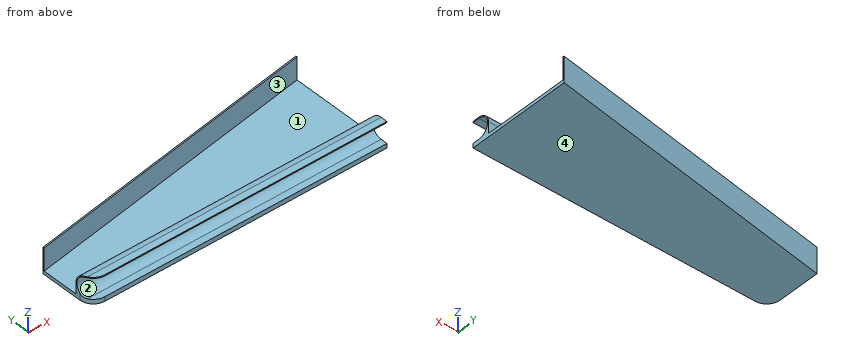
```python
from build123d import *

# Parameters (mm, degrees)
BOSS_EXTRUDE1_DEPTH     = 6.35
BOSS_EXTRUDE7_DEPTH     = 558.8
CUT_EXTRUDE1_DEPTH      = 551.191074589
CUT_EXTRUDE1_DEPTH_BACK = 551.191074589
BOSS_EXTRUDE8_DEPTH     = 42.164
CUT_EXTRUDE2_DEPTH      = 110.49


with BuildPart() as part:
    # Sketch1 → Boss-Extrude1 (new body)
    with BuildSketch(Plane.XY):
        with BuildLine():
            Line((-508.085110878, -34.117945662), (-508.085110878, -168.737945662))
            Line((-508.085110878, -168.737945662), (-508.085110878, -181.437945662))
            ThreePointArc((-508.085110878, -181.437945662), (-500.64562312, -199.398457904), (-482.685110878, -206.837945662))
            Line((-482.685110878, -206.837945662), (50.714889122, -206.837945662))
            Line((50.714889122, -206.837945662), (50.714889122, -8.717945662))
            Line((50.714889122, -8.717945662), (-482.685110878, -8.717945662))
            ThreePointArc((-482.685110878, -8.717945662), (-500.64562312, -16.15743342), (-508.085110878, -34.117945662))
        make_face()
    extrude(amount=BOSS_EXTRUDE1_DEPTH)

    # Sketch3 → Boss-Extrude7 (add)
    with BuildSketch(Plane(origin=(50.714889122, 0, 0), x_dir=(0, 0, -1), z_dir=(1, 0, 0))):
        with BuildLine():
            Line((-6.35, -173.055945662), (-27.432, -173.055945662))
            ThreePointArc((-27.432, -173.055945662), (-42.339225161, -179.230720501), (-48.514, -194.137945662))
            Line((-48.514, -194.137945662), (-48.514, -206.837945662))
            Line((-48.514, -206.837945662), (-46.482, -206.837945662))
            Line((-46.482, -206.837945662), (-46.482, -194.137945662))
            ThreePointArc((-46.482, -194.137945662), (-27.432, -175.087945662), (-8.382, -194.137945662))
            Line((-8.382, -194.137945662), (-8.382, -206.837945662))
            Line((-8.382, -206.837945662), (-6.35, -206.837945662))
            Line((-6.35, -206.837945662), (-6.35, -173.055945662))
        make_face()
    extrude(amount=-BOSS_EXTRUDE7_DEPTH)

    # Sketch4 → Cut-Extrude1 (cut, two sides: drawn at the far end of the back side and taken through both)
    with BuildSketch(Plane.XY.offset(6.35).offset(-CUT_EXTRUDE1_DEPTH_BACK)):
        Polygon((-508.085110878, -101.427945662), (50.714889122, -8.717945662), (-523.466542696, -8.717945662), align=None)
    extrude(amount=CUT_EXTRUDE1_DEPTH + CUT_EXTRUDE1_DEPTH_BACK, mode=Mode.SUBTRACT)

    # Sketch5 → Boss-Extrude8 (add, through all)
    with BuildSketch(Plane.XY.offset(6.35)):
        Polygon((-508.085110878, -101.427945662), (50.714889122, -8.717945662), (50.714889122, -11.257945662), (-508.085110878, -103.967945662), align=None)
    extrude(amount=BOSS_EXTRUDE8_DEPTH)

    # Sketch6 → Cut-Extrude2 (cut)
    with BuildSketch(Plane(origin=(0, 0, 6.35), x_dir=(-1, 0, 0), z_dir=(0, 0, -1))):
        with BuildLine():
            Line((482.685110878, -206.837945662), (508.085110878, -206.837945662))
            Line((508.085110878, -206.837945662), (508.085110878, -181.437945662))
            ThreePointArc((508.085110878, -181.437945662), (500.64562312, -199.398457904), (482.685110878, -206.837945662))
        make_face()
    extrude(amount=-CUT_EXTRUDE2_DEPTH, mode=Mode.SUBTRACT)


solid = part.part
```
Part model, mm, in its own coordinate system. Face numbers are marked on the shaded views. Give positions to 0.01 mm unless a question says otherwise; leave off trailing zeros. Write each loop counter-clockwise with the first axis right and the second up, starting at its lowest first coordinate (ties: lowest second). Pieces come first, ordered by that corner, then holes. Notation, with made-up numbers: (62.25, 83.25) -> (98.25, 83.25) arc R30 cw to (98.25, 105.25) -> close; hole circle Ø3 at (68, 81). An arc over 180 degrees is marked (long way). Put each result on its own line as item: value. Start each with the question number.
Item 1: Pin check, flat tips, straight feed: pin 1 Ø1 at (x, y) = (-107.5, -146) entering from +Z; pin 2 Ø6 at (x, z) = (-226.5, 35.5) entering from +Y; pin 3 Ø23 at (x, z) = (-157, 17) entering from +Y. Stop position of each tip, or through.
Item 2: Pull direction Y, two halves, no side cores. Call the marked faces 1, 2, 3 and 4: pulls with the +Y half, pulls with the -Y half, needs draft (parallel to the pull), parting line crosses it, or undercut.
Item 3: Wall check: L1, parallel to Z at x = -144.5, y = -119; L2, parallel to Z at x = -109.5, y = -197; L3, parallel to Y at x = -364.5, z = 44. Give the ranges that are in metal, low to high. Write a range as [from, to].
Item 4: Cut at B-B (x = -326). List the corners of the cut face in (y, z), then the cut area to 3 significant figures.
Item 5: Cut at D-D (x = -400). List the corners of the cut face in (y, z).
Item 6: Cut at C-C (y = -121.5). List the corners of the cut face in (x, z), then the cut area to 3 significant figures.
Item 7: Cut at A-A (z = 22.5). List the corners of the cut face in (x, y).
Answer list:
1. pin 1: stops at z = 6.35
1. pin 2: stops at y = -54.21
1. pin 3: stops at y = -41.27
2. face 1: undercut
2. face 2: pulls with the -Y half
2. face 3: undercut
2. face 4: needs draft
3. L1: z = [0, 6.35]
3. L2: z = [0, 8.38], [46.48, 48.51]
3. L3: y = [-184.74, -181.1], [-80.15, -77.61]
4. outline: (-206.84, 0) -> (-71.22, 0) -> (-71.22, 48.51) -> (-73.76, 48.51) -> (-73.76, 6.35) -> (-173.06, 6.35) -> (-173.06, 27.43) arc R21.08 ccw to (-194.14, 48.51) -> (-206.84, 48.51) -> (-206.84, 46.48) -> (-194.14, 46.48) arc R19.05 cw to (-194.14, 8.38) -> (-206.84, 8.38) -> close
4. area: 1,240 mm2
5. outline: (-206.84, 0) -> (-83.5, 0) -> (-83.5, 48.51) -> (-86.04, 48.51) -> (-86.04, 6.35) -> (-173.06, 6.35) -> (-173.06, 27.43) arc R21.08 ccw to (-194.14, 48.51) -> (-206.84, 48.51) -> (-206.84, 46.48) -> (-194.14, 46.48) arc R19.05 cw to (-194.14, 8.38) -> (-206.84, 8.38) -> close
6. outline: (-508.09, 0) -> (50.71, 0) -> (50.71, 6.35) -> (-508.09, 6.35) -> close
6. area: 3,550 mm2
7. outline: (-508.09, -175.74) -> (50.71, -175.74) -> (50.71, -173.06) -> (-508.09, -173.06) -> close; (-508.09, -103.97) -> (50.71, -11.26) -> (50.71, -8.72) -> (-508.09, -101.43) -> close
